The drawing under review shows one solid part. Ordinate dimensions are in mm from its lowest x, y, z. A direction names the side the tool comes from. Give positions to 0.01 mm unless a question says otherwise; leave off trailing zeros. Loops run counter-clockwise (first coordinate to the right, second up) from the corner with the lowest first, then second, coordinate; pieces in that order, holes last. Notation, with made-up numbers: M 71,48 L 126,48 A11 cw 126,57 Z; hole C -1.5,23 d4. An arc over 180 degrees is marked long. Answer as CSV lines item,"result".
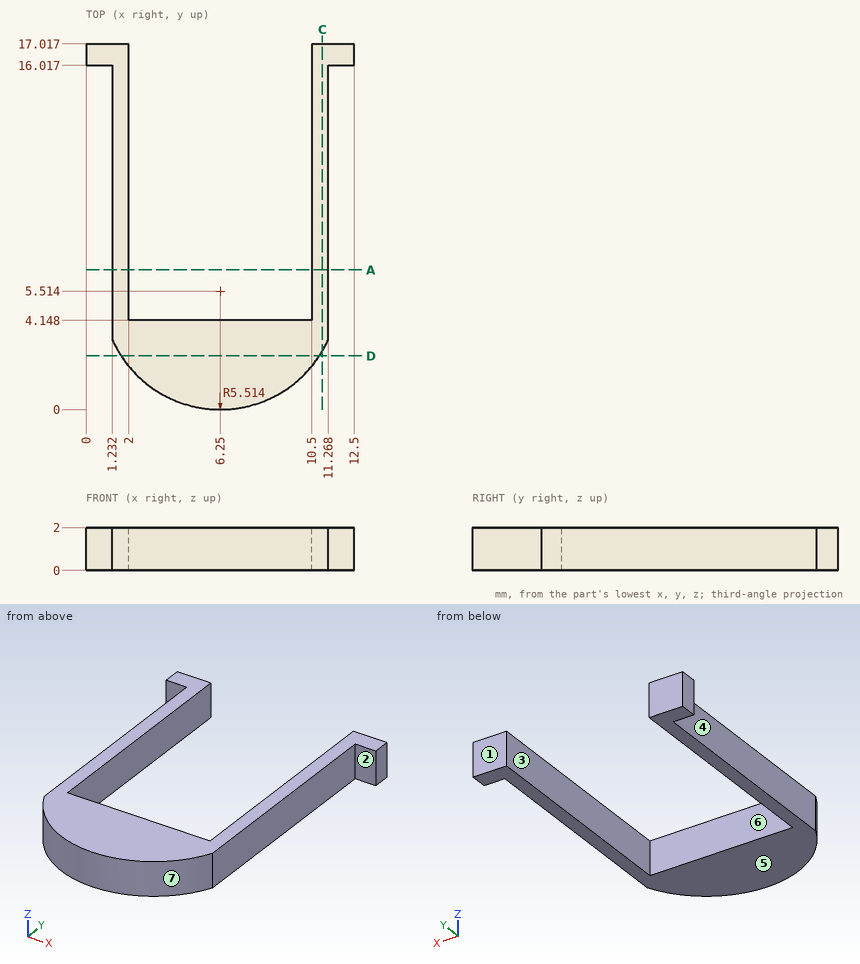
1. We need section D-D, the plane y = 2.5. Write out the cut boundary in (x, z).
Answer block:
outline,"M 1.63,0 L 10.87,0 L 10.87,2 L 1.63,2 Z"
2. The part is to be moulded in two halves that separate along X. For the marked faces 5, 6 and 7, say which applies: pulls with the +X half, pulls with the -X half, needs draft (parallel to the pull), parting line crosses it, or undercut.
Answer block:
face 5,"needs draft"
face 6,"undercut"
face 7,"parting line crosses it"
3. To check wall thickness, follow L1, parallel to X at y = 13, z = 1.8; L2, parallel to X at y = 4, z = 0.1; L3, parallel to X at y = 2, z = 0.45. State the ranges of each line that lie inside material, in increasing order. Write a range as [from, to].
Answer block:
L1,"[1.23, 2], [10.5, 11.27]"
L2,"[1.23, 11.27]"
L3,"[2, 10.5]"
4. For P1, Ø1, axis at x = 3.5, z = 0.5, coming from the -Y side; P2, Ø1, axis at x = 0.5, z = 0.5, coming from the -Y side; P3, Ø1, axis at y = 7.5, z = 1, coming from the +X side, all flat-tipped, find the tip position at first contact; note any pin that passes through.
Answer block:
P1,"y = 0.48"
P2,"y = 16.02"
P3,"x = 11.27"
5. We need section A-A, the plane y = 6.5. Write out the cut boundary in (x, z).
Answer block:
outline,"M 1.23,0 L 2,0 L 2,2 L 1.23,2 Z; M 10.5,0 L 11.27,0 L 11.27,2 L 10.5,2 Z"
6. We need section C-C, the plane x = 11. Write out the cut boundary in (y, z), plus the area to 3 significant figures.
Answer block:
outline,"M 2.71,0 L 17.02,0 L 17.02,2 L 2.71,2 Z"
area,"28.6 mm²"
7. For the marked faces 1, 2, 3 and 4, list the 3-axis set-ups (+Z, -Z, +X, -X, +Y, -Y) from which the entire face can be reached by the end or side of a thin tool; tool diameter is ignored.
Answer block:
face 1,"+Z, -Z, +X, -X, +Y"
face 2,"+Z, -Z, +X, -Y"
face 3,"+Z, -Z, +Y"
face 4,"+Z, -Z, -X, -Y"
